from build123d import *

# Parameters (mm, degrees)
SKETCH1_R               = 2.38125
BOSS_EXTRUDE1_DEPTH     = 9.525
CUT_EXTRUDE3_DEPTH      = 24.599884136
CUT_EXTRUDE3_DEPTH_BACK = 24.599884136
SKETCH5_R               = 2.38125
FILLET1_R               = 4.7625
FILLET2_R               = 3.175
CHAMFER1_SIZE           = 0.396875


with BuildPart() as part:
    # Sketch1 → Boss-Extrude1 (new body)
    with BuildSketch(Plane(origin=(0, 0, 0), x_dir=(1, 0, 0), z_dir=(0, 1, 0))):
        with BuildLine():
            Line((-1.5875, -17.4625), (-1.5875, -6.148361062))
            ThreePointArc((-1.5875, -6.148361062), (-3.888564967, 5.020115786), (6.35, 0))
            Line((6.35, 0), (6.35, -17.4625))
            Line((6.35, -17.4625), (-1.5875, -17.4625))
        make_face()
        with Locations(Location((0, 0, 0), (0, 0, 90))):
            Circle(SKETCH1_R, mode=Mode.SUBTRACT)
    extrude(amount=BOSS_EXTRUDE1_DEPTH)

    # Sketch5 → Cut-Extrude3 (cut, two sides: drawn at the far end of the back side and taken through both)
    with BuildSketch(Plane(origin=(6.35, 0, 0), x_dir=(0, 0, -1), z_dir=(1, 0, 0)).offset(-CUT_EXTRUDE3_DEPTH_BACK)):
        with Locations((-12.7, 4.7625)):
            Circle(SKETCH5_R)
    extrude(amount=CUT_EXTRUDE3_DEPTH + CUT_EXTRUDE3_DEPTH_BACK, mode=Mode.SUBTRACT)

    # Fillet1
    fillet1_edges = [part.edges().sort_by_distance(p)[0] for p in [
        (2.38125, 0, 17.4625),
        (2.38125, 9.525, 17.4625),
    ]]
    fillet(fillet1_edges, radius=FILLET1_R - 0.0001)  # a hair under: the kernel refuses the full size

    # Fillet2
    fillet2_edges = [part.edges().sort_by_distance(p)[0] for p in [
        (-1.5875, 4.7625, 6.148361062),
    ]]
    fillet(fillet2_edges, radius=FILLET2_R)

    # Chamfer1
    chamfer1_edges = [part.edges().sort_by_distance(p)[0] for p in [
        (0, 0, 2.38125),
        (0, 9.525, 2.38125),
        (-3.175, 9.525, -5.499261314),
        (-1.5875, 4.7625, 15.08125),
        (6.35, 4.7625, 15.08125),
        (6.35, 0, 6.35005),
        (6.35, 9.525, 6.35005),
        (6.35, 8.130125335, 16.067625335),
        (6.35, 1.394874665, 16.067625335),
        (-1.5875, 8.130125335, 16.067625335),
        (-1.5875, 1.394874665, 16.067625335),
        (-1.5875, 0, 10.474495986),
        (-1.5875, 9.525, 10.474495986),
        (-2.012869343, 0, 6.661391971),
        (-2.012869343, 9.525, 6.661391971),
        (-3.175, 0, -5.499261314),
    ]]
    chamfer(chamfer1_edges, length=CHAMFER1_SIZE)


solid = part.part
For this review, take the finished solid that the model builds, in its own axes (mm). Give positions to 0.01 mm unless a question says otherwise; leave off trailing zeros. Put each result on its own line as item: value. Start each with the question number.
(1) Wall thickness on L1, parallel to X at y = 2.5, z = 0; L2, parallel to Z at x = 1.5, y = 6; L3, parallel to Y at x = 2.5, z = 12.7 (3 decimals): over which ranges is each line inside the solid? List them lowest first.
(2) The part is to be moulded in two halves that separate along Z. For faces 1 (the cylindrical face through (1.45, 4.7, 1.89)), 2 (the cylindrical face through (2.33, 2.65, 11.6)), 3 (the flat face through (-1.588, 6, 10)), 4 (the conical face through (6.24, 7.96, 15.83)), say which applies: +Z half, -Z half, draft (parallel to the pull), parting line (faces both ways), or undercut.
(3) Add section A-A, the plane x = 0. Give the number of separate pieces and of enclosed holes in the cut face, then the cut area to 3 significant figures.
(4) For pin 1 (1 mm diameter, centred on y = 3.5, z = -3, fed in from -X); pin 2 (1.5 mm diameter, centred on y = 8.5, z = -3, fed in from -X); pin 3 (1.5 mm diameter, centred on y = 7, z = 1, fed in from -X), all flat-tipped, find the tip position at first contact; note any pin that passes through.
Result:
1. L1: x = -6.35 to -2.38, 2.38 to 6.35
1. L2: z = -6.17 to -1.85, 1.85 to 10.67, 14.73 to 17.3
1. L3: y = 0 to 2.381, 7.144 to 9.525
2. face 1: undercut
2. face 2: undercut
2. face 3: draft
2. face 4: +Z half
3. separate pieces: 2
3. enclosed holes: 1
3. area: 153 mm^2
4. pin 1: stops at x = -5.84
4. pin 2: stops at x = -5.94
4. pin 3: stops at x = -6.35
